Can you work these out from the model? Positions are in its coordinate system, mm. Give positions to 0.01 mm unless a question says otherwise; leave off trailing zeros. Write each loop counter-clockwise with the first axis right and the second up, starting at its lowest first coordinate (ties: lowest second). Pieces come first, ordered by that corner, then holes.
1. Suppose I cut it at A-A (y = -110.5). Please give me the cut outline in (x, z), and give its area (3 significant figures).
2. Suppose I cut it at B-B (x = -47). Please give me the cut outline in (y, z).
3. I'm going to push flat-ended pins straight in: pin 1 (1 mm diameter, centred on x = 37.5, z = 25.5, fed in from -Y); pin 2 (1 mm diameter, centred on x = -63, z = 11.5, fed in from -Y); pin 3 (1 mm diameter, centred on y = 28.5, z = 32, fed in from +X); pin 4 (1.5 mm diameter, centred on x = 66, y = -59.5, fed in from -Z). Where does each tip first touch, or does it pass through?
4. Suppose I cut it at C-C (z = 40.5). Please give me the cut outline in (x, y), and give its area (3 significant figures).
5. If I drill on probe 1 along Y at (x, z) = (-30.5, 32); probe 2 along Y at (x, z) = (-31, 25); probe 3 along X at (y, z) = (-45, 18.5), over which ranges is the centre line in solid material (lowest first)?
```python
from build123d import *

# Parameters (mm, degrees)
F1_DEPTH   = 49.276
F1_FACE_W  = 39.7166078589
F1_FACE_H  = 49.276
F1_FACE1_W = 89.1782223892
F1_FACE1_H = 49.276


with BuildPart() as f1:
    # F0 (on Top) → F1 (new body)
    with BuildSketch(Plane.XY):
        Polygon((28.3779297024, 27.7867242694), (0, 55.5734485388), (0, -56.7558594048), align=None)
    extrude(amount=F1_DEPTH)

    # F1_face (on face) → F2 (revolve)
    with BuildSketch(Plane(origin=(14.1889648512, 41.6800864041, 24.638), x_dir=(-0.7145104084, 0.6996248111, 0), z_dir=(0.6996248111, 0.7145104084, 0))):
        Rectangle(F1_FACE_W, F1_FACE_H)
    revolve(axis=Axis((0, 55.5734485388, 24.638), (0, 0, -1)))

    # F1_face1 (on face) → F3 (revolve)
    with BuildSketch(Plane(origin=(14.1889648512, -14.4845675677, 24.638), x_dir=(0.3182159157, 0.9480182651, 0), z_dir=(0.9480182651, -0.3182159157, 0))):
        Rectangle(F1_FACE1_W, F1_FACE1_H)
    revolve(axis=Axis((0, -56.7558594048, 24.638), (0, 0, -1)))


solid = f1.part
```
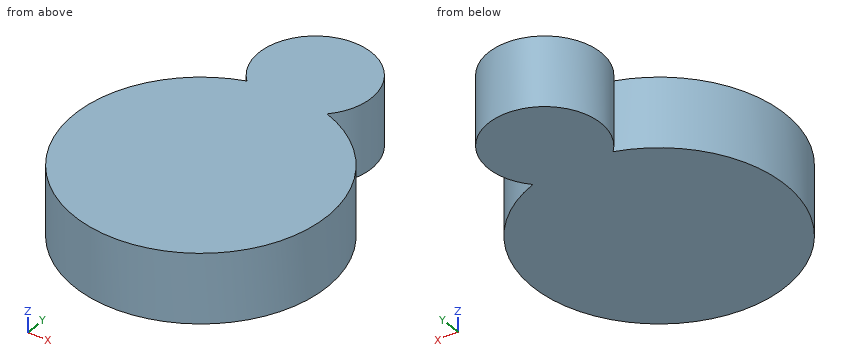
Checks:
1. outline: (-71.16, 0) - (71.16, 0) - (71.16, 49.28) - (-71.16, 49.28) - close
1. area: 7,010 mm2
2. outline: (-132.54, 0) - (19.03, 0) - (19.03, 49.28) - (-132.54, 49.28) - close
3. pin 1: stops at y = -137.9
3. pin 2: stops at y = -120.37
3. pin 3: stops at x = 29.52
3. pin 4: stops at z = 0
4. outline: (-28.38, 27.79) arc R89.18 ccw (long way) to (28.38, 27.79) arc R39.72 ccw (long way) to start
4. area: 29,300 mm2
5. probe 1: y = -140.56 to 27.04, 30.13 to 81.01
5. probe 2: y = -140.37 to 26.86, 30.75 to 80.4
5. probe 3: x = -88.4 to 88.4
